from build123d import *

# Parameters (mm, degrees)
F2_DEPTH = 4.5
F0_R     = 3.1
F3_DEPTH = 4.501
F0_W     = 39.4
F0_H     = 16.4
F4_DEPTH = 3.5
F5_R     = 2
F6_R     = 5


with BuildPart() as f2:
    # F1 (on Top) → F2 (new body)
    with BuildSketch(Plane.XY):
        with BuildLine():
            Line((-21.2, -1.8), (-15.328208, -1.8))
            ThreePointArc((-15.328208, -1.8), (-15.082723, -0.914839), (-15, 0))
            ThreePointArc((-15, 0), (-23.293744, 3.976179), (-21.2, -4.97996))
            Line((-21.2, -4.97996), (-21.2, -1.8))
        make_face()
        with BuildLine():
            ThreePointArc((21.2, -4.97996), (17.671307, -4.484579), (15.328208, -1.8))
            Line((15.328208, -1.8), (-15.328208, -1.8))
            ThreePointArc((-15.328208, -1.8), (-17.671307, -4.484579), (-21.2, -4.97996))
            Line((-21.2, -4.97996), (-21.2, -21.2))
            Line((-21.2, -21.2), (21.2, -21.2))
            Line((21.2, -21.2), (21.2, -4.97996))
        make_face()
        with BuildLine():
            Line((15.328208, -1.8), (21.2, -1.8))
            Line((21.2, -1.8), (21.2, -4.97996))
            ThreePointArc((21.2, -4.97996), (24.076179, -3.193744), (25.2, 0))
            ThreePointArc((25.2, 0), (19.185161, 5.017277), (15.328208, -1.8))
        make_face()
        with BuildLine():
            Line((21.2, -4.97996), (21.2, -1.8))
            Line((21.2, -1.8), (15.328208, -1.8))
            ThreePointArc((15.328208, -1.8), (17.671307, -4.484579), (21.2, -4.97996))
        make_face()
        with BuildLine():
            ThreePointArc((-21.2, -4.97996), (-17.671307, -4.484579), (-15.328208, -1.8))
            Line((-15.328208, -1.8), (-21.2, -1.8))
            Line((-21.2, -1.8), (-21.2, -4.97996))
        make_face()
    extrude(amount=-F2_DEPTH)

    # F0 (on Top) → F3 (cut, through all)
    with BuildSketch(Plane.XY):
        with Locations((-20.1, 0)):
            Circle(F0_R)
        with BuildLine():
            ThreePointArc((23.2, 0), (20.1, 3.1), (17, 0))
            ThreePointArc((17, 0), (20.1, -3.1), (23.2, 0))
        make_face()
    extrude(amount=-F3_DEPTH, mode=Mode.SUBTRACT)

    # F0 (on Top) → F4 (cut)
    with BuildSketch(Plane.XY):
        with Locations((0, -11.5)):
            Rectangle(F0_W, F0_H)
    extrude(amount=-F4_DEPTH, mode=Mode.SUBTRACT)

    # F5
    f5_edges = [f2.edges().sort_by_distance(p)[0] for p in [
        (-21.2, -21.2, -2.25),
        (21.2, -21.2, -2.25),
    ]]
    fillet(f5_edges, radius=F5_R)

    # F6
    f6_edges = [f2.edges().sort_by_distance(p)[0] for p in [
        (-21.2, -4.97996, -2.25),
        (-15.328208, -1.8, -2.25),
        (21.2, -4.97996, -2.25),
        (15.328208, -1.8, -2.25),
    ]]
    fillet(f6_edges, radius=F6_R)


solid = f2.part
Here's how the part is built. I have some questions about the finished solid (model axes, mm). A direction names the side the tool comes from. Coordinates: 2 decimals unless noted, no trailing zeros. Order: outer loops, then holes, each group sorted by start corner. A loop starts at its lowest first (then second) coordinate and runs counter-clockwise, first axis right, second up. Notation, with made-up numbers: (-30, -0.75) - (-10, -0.75) arc R22 cw to (-10, 18.25) - close; hole circle Ø6 at (73.5, 22). An arc over 180 degrees is marked (long way). Use CSV: the item, a comma, the result in double quotes. Start each with the question number.
1. I'm going to push flat-ended pins straight in: pin 1 (5 mm diameter, centred on x = -20.1, y = 0, fed in from +Z); pin 2 (1.8 mm diameter, centred on y = -11.5, z = -1.5, fed in from -X); pin 3 (2 mm diameter, centred on y = -14.5, z = -3, fed in from +X). Where does each tip first touch, or does it pass through?
2. If we mould it in two halves opening along X, with no side actions, what happens to faces 1 (the face through (0, -19.7, -2)), 2 (the face through (-21.2, -14, -2)), 3 (the face through (0, -11, -4.5))? For each: +X half, -X half, draft (parallel to the pull), parting line (faces both ways), or undercut.
3. Suppose I cut it at C-C on z = -0.7. Give the number of separate pieces and of enclosed holes in the cut face, then the cut area to 3 significant figures.
4. Please list where these lines run through material, in increasing order: line 1 (X direction, y = -8.75, z = -1.05); line 2 (Y direction, x = -9, z = -0.7); line 3 (Y direction, x = 18.5, z = -1.3). Write a range as from..to.
5. Suppose I cut it at D-D on x = 6. List the corners of the cut face in (y, z) for me.
6. Suppose I cut it at B-B on y = -10.25. List the corners of the cut face in (x, z) for me.
7. Suppose I cut it at A-A on x = 17.5. List the corners of the cut face in (y, z) for me.
8. For faces 4 (the face through (21.2, -14, -2)), 5 (the face through (0, -3, 0)), 6 (the face through (0, -1.8, -2)), 7 (the face through (-19.7, -12, -2)), which set-ups out of +Z, -Z, +X, -X, +Y, -Y let a thin tool reach every point of the face, with its end or its side?
Output:
1,pin 1,"passes through"
1,pin 2,"stops at x = -21.2"
1,pin 3,"stops at x = 21.2"
2,face 1,"undercut"
2,face 2,"-X half"
2,face 3,"draft"
3,separate pieces,"1"
3,enclosed holes,"3"
3,area,"258 mm2"
4,line 1,"x = -21.2..-19.7, 19.7..21.2"
4,line 2,"y = -21.2..-19.7, -3.3..-1.8"
4,line 3,"y = -21.2..-19.7, -3.3..-2.66, 2.66..4.84"
5,outline,"(-21.2, -4.5) - (-1.8, -4.5) - (-1.8, 0) - (-3.3, 0) - (-3.3, -3.5) - (-19.7, -3.5) - (-19.7, 0) - (-21.2, 0) - close"
6,outline,"(-21.2, -4.5) - (21.2, -4.5) - (21.2, 0) - (19.7, 0) - (19.7, -3.5) - (-19.7, -3.5) - (-19.7, 0) - (-21.2, 0) - close"
7,outline,"(-21.2, -4.5) - (-1.69, -4.5) - (-1.69, 0) - (-3.3, 0) - (-3.3, -3.5) - (-19.7, -3.5) - (-19.7, 0) - (-21.2, 0) - close; (1.69, -4.5) - (4.39, -4.5) - (4.39, 0) - (1.69, 0) - close"
8,face 4,"+Z, -Z, +X, -Y"
8,face 5,"+Z, +X, -X, +Y, -Y"
8,face 6,"+Z, -Z, +Y"
8,face 7,"+Z"
